Could you check a few things on this model? Use its own coordinates, in mm. A direction names the side the tool comes from. Coordinates: 2 decimals unless noted, no trailing zeros. Order: outer loops, then holes, each group sorted by start corner. A loop starts at its lowest first (then second) coordinate and runs counter-clockwise, first axis right, second up. Notation, with made-up numbers: (42.5, 71) - (100.5, 71) arc R23 cw to (100.5, 87) - close; hole circle Ø1 at (47, 79.5). An arc over 180 degrees is marked (long way). One line per item, written item: value.
from build123d import *

# Parameters (mm, degrees)
F0_R     = 4.25
F1_DEPTH = 100


# Not quite as in the source:
# - a feature of the source that left no trace in its solid (it failed there, or was rolled back) is left out


with BuildPart() as f1:
    # F0 (on Front) → F1 (new body)
    with BuildSketch(Plane.XZ):
        Circle(F0_R)
        with BuildLine():
            ThreePointArc((2.265, 2.1737237635), (2.8140381057, 1.6246856578), (3.015, 0.8746856578))
            Line((3.015, 0.8746856578), (3.015, -0.8746856578))
            ThreePointArc((3.015, -0.8746856578), (2.8140381057, -1.6246856578), (2.265, -2.1737237635))
            Line((2.265, -2.1737237635), (0.75, -3.0484094213))
            ThreePointArc((0.75, -3.0484094213), (0, -3.2493713156), (-0.75, -3.0484094213))
            Line((-0.75, -3.0484094213), (-2.265, -2.1737237635))
            ThreePointArc((-2.265, -2.1737237635), (-2.8140381057, -1.6246856578), (-3.015, -0.8746856578))
            Line((-3.015, -0.8746856578), (-3.015, 0.8746856578))
            ThreePointArc((-3.015, 0.8746856578), (-2.8140381057, 1.6246856578), (-2.265, 2.1737237635))
            Line((-2.265, 2.1737237635), (-0.75, 3.0484094213))
            ThreePointArc((-0.75, 3.0484094213), (0, 3.2493713156), (0.75, 3.0484094213))
            Line((0.75, 3.0484094213), (2.265, 2.1737237635))
        make_face(mode=Mode.SUBTRACT)
    extrude(amount=F1_DEPTH)


solid = f1.part
Item 1: I'm going to push flat-ended pins straight in: pin 1 Ø1.5 at (x, y) = (1.5, -71.5) entering from +Z; pin 2 Ø1.5 at (y, z) = (-53.5, -1) entering from -X. Where does each tip first touch, or does it pass through?
Conclusion:
pin 1: z = 4.18
pin 2: x = -4.24
Item 2: If I drill on probe 1 along Z at (x, y) = (-0.25, -82.5); probe 2 along Z at (x, y) = (-0.75, -41); probe 3 along X at (y, z) = (-50, -1.75), over which ranges is the centre line in solid material (lowest first)?
Conclusion:
probe 1: -4.24 to -3.23, 3.23 to 4.24
probe 2: -4.18 to -3.05, 3.05 to 4.18
probe 3: -3.87 to -2.73, 2.73 to 3.87
Item 3: For faces 1 (the face through (-3.2, -100, 0)), 2 (the face through (1.497, -49.3, 2.617)), which set-ups out of +Z, -Z, +X, -X, +Y, -Y let a thin tool reach every point of the face, with its end or its side?
Conclusion:
face 1: +Z, -Z, +X, -X, -Y
face 2: +Y, -Y
Item 4: I want a section at B-B on y = -53.5. Please give me the cut outline in (x, z) (3 decimals), then the cut area to 3 significant figures.
Conclusion:
outline: circle Ø8.5 at (0, 0); hole (-3.015, -0.875) arc R1.5 ccw to (-2.265, -2.174) - (-0.75, -3.048) arc R1.5 ccw to (0.75, -3.048) - (2.265, -2.174) arc R1.5 ccw to (3.015, -0.875) - (3.015, 0.875) arc R1.5 ccw to (2.265, 2.174) - (0.75, 3.048) arc R1.5 ccw to (-0.75, 3.048) - (-2.265, 2.174) arc R1.5 ccw to (-3.015, 0.875) - close
area: 26.0 mm²
Item 5: Thinking about a two-plate mould opening in Z: for faces 3 (the face through (2.285, -49.3, 3.584)), 4 (the face through (-3.2, 0, 0)), 5 (the face through (-3.015, -49, 0)), which applies, pulls with the +Z half, pulls with the -Z half, needs draft (parallel to the pull), parting line crosses it, or undercut?
Conclusion:
face 3: parting line crosses it
face 4: needs draft
face 5: undercut
Item 6: I want a section at A-A on z = 0. Please give me the cut outline in (x, y) (3 decimals), then the cut area to 3 significant figures.
Conclusion:
outline: (-4.25, -100) - (-3.015, -100) - (-3.015, 0) - (-4.25, 0) - close; (3.015, -100) - (4.25, -100) - (4.25, 0) - (3.015, 0) - close
area: 247 mm²
